Read the model definition and answer for the solid it produces. Units are mm, in the model's axes. Coordinates: 2 decimals unless noted, no trailing zeros. Order: outer loops, then holes, each group sorted by start corner. A loop starts at its lowest first (then second) coordinate and runs counter-clockwise, first axis right, second up. Notation, with made-up numbers: (-21, 46.25) -> (-13, 46.25) arc R22 ccw to (-13, 62.25) -> close; hole circle Ø11 at (11.25, 87). An arc over 180 degrees is marked (long way). Answer as a JSON object with one key per item and string values. Group by question number.
1) Section A-A on y = 2 is taken. Count the separate pieces of the cut face and the enclosed holes in it, and give its area (3 significant figures).
2) Consider L1, parallel to Y at x = 4.75, z = 23; L2, parallel to Y at x = 0.75, z = -68; L3, parallel to Y at x = 6.5, z = 73. Determine where each line is inside the solid, lowest interval first.
3) Given pin 1 (3 mm diameter, centred on x = 6, y = -15.5, fed in from -Z); pin 2 (3 mm diameter, centred on x = 6.5, z = -79.5, fed in from -Y); pin 3 (8 mm diameter, centred on y = -29, z = -57.5, fed in from -X); pin 4 (2 mm diameter, centred on x = 6.5, y = 23, fed in from +Z), each flat-ended and moving along its own axis, determine where each tip first touches the part or whether it passes through.
4) Section B-B on z = 52.5 is taken. Determine the outline of the cut face in (x, y).
from build123d import *

# Parameters (mm, degrees)
BOSS_EXTRUDE2_DEPTH = 10
CUT_EXTRUDE1_DEPTH  = 10
SKETCH3_W           = 10
SKETCH3_H           = 10
BOSS_EXTRUDE4_DEPTH = 10
SKETCH4_W           = 10
SKETCH4_H           = 10
BOSS_EXTRUDE5_DEPTH = 10
BOSS_EXTRUDE6_REACH = 129.867
SKETCH6_W           = 10
SKETCH6_H           = 10


with BuildPart() as part:
    # Sketch1 → Boss-Extrude2 (new body)
    with BuildSketch(Plane(origin=(0, 0, 0), x_dir=(0, 0, -1), z_dir=(1, 0, 0))):
        with BuildLine():
            Line((-65, 50), (65, 50))
            ThreePointArc((65, 50), (72.071067812, 47.071067812), (75, 40))
            Line((75, 40), (75, -40))
            ThreePointArc((75, -40), (72.071067812, -47.071067812), (65, -50))
            Line((65, -50), (-65, -50))
            ThreePointArc((-65, -50), (-72.071067812, -47.071067812), (-75, -40))
            Line((-75, -40), (-75, 40))
            ThreePointArc((-75, 40), (-72.071067812, 47.071067812), (-65, 50))
        make_face()
    extrude(amount=BOSS_EXTRUDE2_DEPTH)

    # Sketch2 → Cut-Extrude1 (cut)
    with BuildSketch(Plane(origin=(10, 0, 0), x_dir=(0, 0, -1), z_dir=(1, 0, 0))):
        with BuildLine():
            Line((-70, 40), (-70, -40))
            ThreePointArc((-70, -40), (-68.535533906, -43.535533906), (-65, -45))
            Line((-65, -45), (65, -45))
            ThreePointArc((65, -45), (68.535533906, -43.535533906), (70, -40))
            Line((70, -40), (70, 40))
            ThreePointArc((70, 40), (68.535533906, 43.535533906), (65, 45))
            Line((65, 45), (-65, 45))
            ThreePointArc((-65, 45), (-68.535533906, 43.535533906), (-70, 40))
        make_face()
    extrude(amount=-CUT_EXTRUDE1_DEPTH, mode=Mode.SUBTRACT)

    # Sketch3 → Boss-Extrude4 (add)
    with BuildSketch(Plane.XY.offset(75)):
        with Locations((5, 35)):
            Rectangle(SKETCH3_W, SKETCH3_H)
        with Locations((5, -35)):
            Rectangle(SKETCH3_W, SKETCH3_H)
    extrude(amount=BOSS_EXTRUDE4_DEPTH)

    # Sketch4 → Boss-Extrude5 (add)
    with BuildSketch(Plane(origin=(0, 0, -75), x_dir=(-1, 0, 0), z_dir=(0, 0, -1))):
        with Locations((-5, 35)):
            Rectangle(SKETCH4_W, SKETCH4_H)
        with Locations((-5, -35)):
            Rectangle(SKETCH4_W, SKETCH4_H)
    extrude(amount=BOSS_EXTRUDE5_DEPTH)

    # Boss-Extrude6: up to this face of the body (flat: up to its plane)
    boss_extrude6_end = Plane(part.part.faces().sort_by_distance((5, 45, 0))[0])
    # Sketch6 → Boss-Extrude6 (add, up to the picked face)
    with BuildSketch(Plane(origin=(0, -45, 0), x_dir=(1, 0, 0), z_dir=(0, 1, 0)), mode=Mode.PRIVATE) as boss_extrude6_sk1:
        with Locations((5, 60)):
            Rectangle(SKETCH6_W, SKETCH6_H)
    boss_extrude6_tool1 = split(extrude(boss_extrude6_sk1.sketch, amount=BOSS_EXTRUDE6_REACH, mode=Mode.PRIVATE), bisect_by=boss_extrude6_end, keep=Keep.BOTH, mode=Mode.PRIVATE)
    # Sketch6 → Boss-Extrude6 (add, up to the picked face)
    with BuildSketch(Plane(origin=(0, -45, 0), x_dir=(1, 0, 0), z_dir=(0, 1, 0)), mode=Mode.PRIVATE) as boss_extrude6_sk2:
        with Locations((5, 36)):
            Rectangle(SKETCH6_W, SKETCH6_H)
    boss_extrude6_tool2 = split(extrude(boss_extrude6_sk2.sketch, amount=BOSS_EXTRUDE6_REACH, mode=Mode.PRIVATE), bisect_by=boss_extrude6_end, keep=Keep.BOTH, mode=Mode.PRIVATE)
    # Sketch6 → Boss-Extrude6 (add, up to the picked face)
    with BuildSketch(Plane(origin=(0, -45, 0), x_dir=(1, 0, 0), z_dir=(0, 1, 0)), mode=Mode.PRIVATE) as boss_extrude6_sk3:
        with Locations((5, 12)):
            Rectangle(SKETCH6_W, SKETCH6_H)
    boss_extrude6_tool3 = split(extrude(boss_extrude6_sk3.sketch, amount=BOSS_EXTRUDE6_REACH, mode=Mode.PRIVATE), bisect_by=boss_extrude6_end, keep=Keep.BOTH, mode=Mode.PRIVATE)
    # Sketch6 → Boss-Extrude6 (add, up to the picked face)
    with BuildSketch(Plane(origin=(0, -45, 0), x_dir=(1, 0, 0), z_dir=(0, 1, 0)), mode=Mode.PRIVATE) as boss_extrude6_sk4:
        with Locations((5, -12)):
            Rectangle(SKETCH6_W, SKETCH6_H)
    boss_extrude6_tool4 = split(extrude(boss_extrude6_sk4.sketch, amount=BOSS_EXTRUDE6_REACH, mode=Mode.PRIVATE), bisect_by=boss_extrude6_end, keep=Keep.BOTH, mode=Mode.PRIVATE)
    # Sketch6 → Boss-Extrude6 (add, up to the picked face)
    with BuildSketch(Plane(origin=(0, -45, 0), x_dir=(1, 0, 0), z_dir=(0, 1, 0)), mode=Mode.PRIVATE) as boss_extrude6_sk5:
        with Locations((5, -60)):
            Rectangle(SKETCH6_W, SKETCH6_H)
    boss_extrude6_tool5 = split(extrude(boss_extrude6_sk5.sketch, amount=BOSS_EXTRUDE6_REACH, mode=Mode.PRIVATE), bisect_by=boss_extrude6_end, keep=Keep.BOTH, mode=Mode.PRIVATE)
    # Sketch6 → Boss-Extrude6 (add, up to the picked face)
    with BuildSketch(Plane(origin=(0, -45, 0), x_dir=(1, 0, 0), z_dir=(0, 1, 0)), mode=Mode.PRIVATE) as boss_extrude6_sk6:
        with Locations((5, -36)):
            Rectangle(SKETCH6_W, SKETCH6_H)
    boss_extrude6_tool6 = split(extrude(boss_extrude6_sk6.sketch, amount=BOSS_EXTRUDE6_REACH, mode=Mode.PRIVATE), bisect_by=boss_extrude6_end, keep=Keep.BOTH, mode=Mode.PRIVATE)
    add(boss_extrude6_tool1.solids().sort_by(Axis((5, -45, -60), (0, 1, 0)))[0])
    add(boss_extrude6_tool2.solids().sort_by(Axis((5, -45, -36), (0, 1, 0)))[0])
    add(boss_extrude6_tool3.solids().sort_by(Axis((5, -45, -12), (0, 1, 0)))[0])
    add(boss_extrude6_tool4.solids().sort_by(Axis((5, -45, 12), (0, 1, 0)))[0])
    add(boss_extrude6_tool5.solids().sort_by(Axis((5, -45, 60), (0, 1, 0)))[0])
    add(boss_extrude6_tool6.solids().sort_by(Axis((5, -45, 36), (0, 1, 0)))[0])


solid = part.part
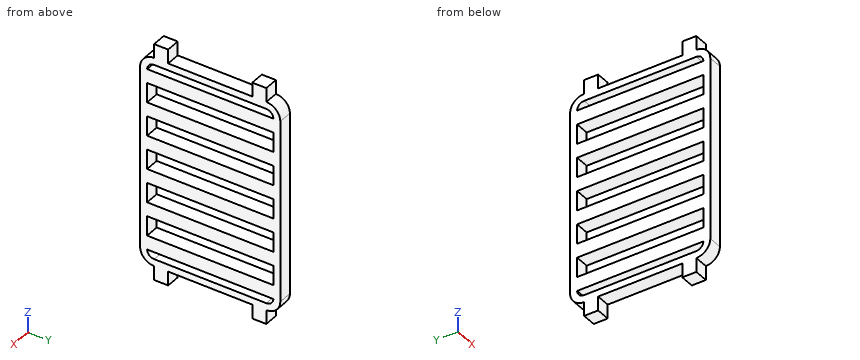
Worked answers:
{
 "1": {"separate pieces": "8", "enclosed holes": "0", "area": "700 mm²"},
 "2": {"L1": "y = -50 to -45, 45 to 50", "L2": "y = -49.54 to -44, 44 to 49.54", "L3": "y = -46 to 46"},
 "3": {"pin 1": "stops at z = -75", "pin 2": "stops at y = -40", "pin 3": "stops at x = 0", "pin 4": "stops at z = 75"},
 "4": {"outline": "(0, -50) -> (10, -50) -> (10, -45) -> (0, -45) -> close; (0, 45) -> (10, 45) -> (10, 50) -> (0, 50) -> close"}
}
